```python
from build123d import *

# Parameters (mm, degrees)
SKETCH001_R = 2.9
PAD_DEPTH   = 70


with BuildPart() as part:
    # Sketch001 → Pad (new body, symmetric)
    with BuildSketch(Plane.XY):
        with BuildLine():
            Line((-8, -3), (-10, -3))
            Line((-10, -3), (-10, -9))
            ThreePointArc((-10, -9), (-9.707107, -9.707107), (-9, -10))
            Line((-9, -10), (-3, -10))
            Line((-3, -10), (-3, -8))
            Line((-3, -8), (-6, -8))
            Line((-6, -8), (-6, -7.06066))
            Line((-6, -7.06066), (-2.93934, -4))
            Line((-2.93934, -4), (-0.65359, -4))
            ThreePointArc((-0.65359, -4), (-0.52418, -3.982963), (-0.40359, -3.933013))
            Line((-0.40359, -3.933013), (0, -3.7))
            Line((0, -3.7), (0.40359, -3.933013))
            ThreePointArc((0.40359, -3.933013), (0.65359, -4), (0.90359, -3.933013))
            Line((0.90359, -3.933013), (1.218886, -3.750977))
            Line((1.218886, -3.750977), (2.5, -4))
            Line((2.5, -4), (2.93934, -4))
            Line((2.93934, -4), (6, -7.06066))
            Line((6, -7.06066), (6, -8))
            Line((6, -8), (3, -8))
            Line((3, -8), (3, -10))
            Line((3, -10), (9, -10))
            ThreePointArc((9, -10), (9.707107, -9.707107), (10, -9))
            Line((10, -9), (10, -3))
            Line((10, -3), (8, -3))
            Line((8, -3), (8, -6))
            Line((8, -6), (7.06066, -6))
            Line((7.06066, -6), (4, -2.93934))
            Line((4, -2.93934), (4, -0.65359))
            ThreePointArc((4, -0.65359), (3.982963, -0.52418), (3.933013, -0.40359))
            Line((3.933013, -0.40359), (3.7, 0))
            Line((3.7, 0), (3.933013, 0.40359))
            ThreePointArc((3.933013, 0.40359), (4, 0.65359), (3.933013, 0.90359))
            Line((3.933013, 0.90359), (3.750977, 1.218886))
            Line((3.750977, 1.218886), (4, 2.5))
            Line((4, 2.5), (4, 2.93934))
            Line((4, 2.93934), (7.06066, 6))
            Line((7.06066, 6), (8, 6))
            Line((8, 6), (8, 3))
            Line((8, 3), (10, 3))
            Line((10, 3), (10, 9))
            ThreePointArc((10, 9), (9.707107, 9.707107), (9, 10))
            Line((9, 10), (3, 10))
            Line((3, 10), (3, 8))
            Line((3, 8), (6, 8))
            Line((6, 8), (6, 7.06066))
            Line((6, 7.06066), (2.93934, 4))
            Line((2.93934, 4), (0.65359, 4))
            ThreePointArc((0.65359, 4), (0.52418, 3.982963), (0.40359, 3.933013))
            Line((0.40359, 3.933013), (0, 3.7))
            Line((0, 3.7), (-0.40359, 3.933013))
            ThreePointArc((-0.40359, 3.933013), (-0.65359, 4), (-0.90359, 3.933013))
            Line((-0.90359, 3.933013), (-1.218886, 3.750977))
            Line((-1.218886, 3.750977), (-2.5, 4))
            Line((-2.5, 4), (-2.93934, 4))
            Line((-2.93934, 4), (-6, 7.06066))
            Line((-6, 7.06066), (-6, 8))
            Line((-6, 8), (-3, 8))
            Line((-3, 8), (-3, 10))
            Line((-3, 10), (-9, 10))
            ThreePointArc((-9, 10), (-9.707107, 9.707107), (-10, 9))
            Line((-10, 9), (-10, 3))
            Line((-10, 3), (-8, 3))
            Line((-8, 3), (-8, 6))
            Line((-8, 6), (-7.06066, 6))
            Line((-7.06066, 6), (-4, 2.93934))
            Line((-4, 2.93934), (-4, 0.65359))
            ThreePointArc((-4, 0.65359), (-3.982963, 0.52418), (-3.933013, 0.40359))
            Line((-3.933013, 0.40359), (-3.7, 0))
            Line((-3.7, 0), (-3.933013, -0.40359))
            ThreePointArc((-3.933013, -0.40359), (-4, -0.65359), (-3.933013, -0.90359))
            Line((-3.933013, -0.90359), (-3.750977, -1.218886))
            Line((-3.750977, -1.218886), (-4, -2.5))
            Line((-4, -2.5), (-4, -2.93934))
            Line((-4, -2.93934), (-7.06066, -6))
            Line((-7.06066, -6), (-8, -6))
            Line((-8, -6), (-8, -3))
        make_face()
        Circle(SKETCH001_R, mode=Mode.SUBTRACT)
    extrude(amount=PAD_DEPTH, both=True)


solid = part.part
```
The model under review builds one solid part; all positions refer to its coordinate system, in mm. A direction names the side the tool comes from. Give positions to 0.01 mm unless a question says otherwise; leave off trailing zeros. Answer in a Markdown table with one row per item. Add a question column.
1. Tool access review of faces 1 (the flat face through (4, -2, 1)), 2 (the flat face through (-4.49, -5.55, 0.98)), 3 (the flat face through (6, -10, 1)), 4 (the flat face through (-10, -6, 1)), 5 (the flat face through (-4, 2, 1)): name each direction out of +Z, -Z, +X, -X, +Y, -Y from which nothing blocks a thin tool from reaching the whole face with its end or side.
2. Insertion check: P1, Ø0.6, axis at x = 9.5, z = -14.5, coming from the +Y side. The pin has a flat end and moves straight along its axis. Give the tip position at first contact, or say it passes through.
3. Wall thickness on line 1 along X through (y, z) = (-4.25, -22); line 2 along X through (y, z) = (7.75, -52.5): over which ranges is each line inside the solid? List them lowest first. Write a range as [from, to].
4. Draft analysis for pull direction X (two halves, no side actions). For faces 6 (the flat face through (-4.45, 5.51, 0.98)), 7 (the flat face through (10, 6, 1)), 8 (the flat face through (2.1, 2.4, 70)), state which applies: +X half, -X half, draft (parallel to the pull), parting line (faces both ways), or undercut.
Ans:
| question | item | result |
|---|---|---|
| 1 | face 1 | +Z, -Z, +X |
| 1 | face 2 | +Z, -Z |
| 1 | face 3 | +Z, -Z, +X, -X, -Y |
| 1 | face 4 | +Z, -Z, -X, +Y, -Y |
| 1 | face 5 | +Z, -Z, -X |
| 2 | P1 | stops at y = 9.98 |
| 3 | line 1 | x = [-10, -8], [-5.31, -3.19], [3.19, 5.31], [8, 10] |
| 3 | line 2 | x = [-10, -6], [6, 10] |
| 4 | face 6 | undercut |
| 4 | face 7 | +X half |
| 4 | face 8 | draft |
